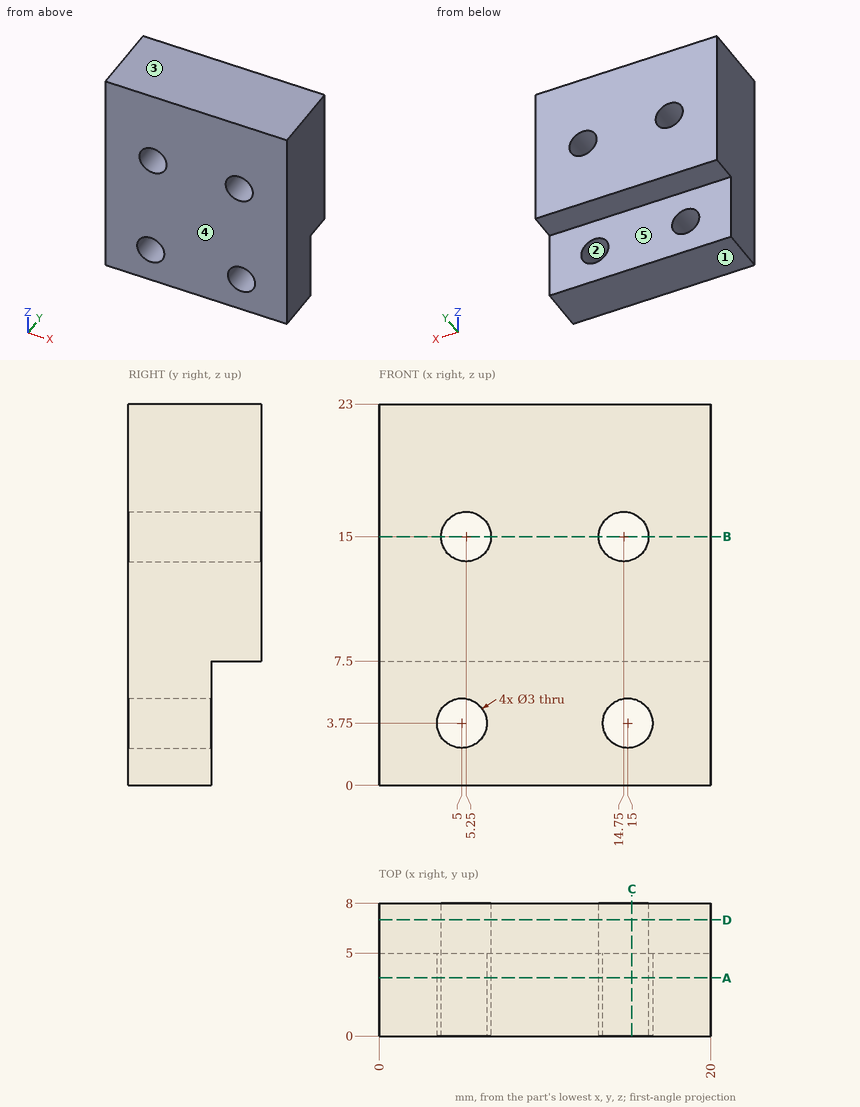
Answer from the drawing. Dimensions are ordinates in mm from the lowest x, y and z of the part. A direction names the side the tool comes from. Coordinates: 2 decimals unless noted, no trailing zeros. Loops run counter-clockwise (first coordinate to the right, second up) from the corner with the lowest first, then second, coordinate; pieces in that order, holes last. Notation, with made-up numbers: (60.25, 29.5) - (78.25, 29.5) arc R14 ccw to (78.25, 34.5) - close; hole circle Ø6 at (-22.5, 83). An arc over 180 degrees is marked (long way). Use a Markdown table: item, result.
Item 1: Find section C-C, the plane x = 15.25. Determine the outline of the cut face in (y, z), and give its area (3 significant figures).
Evaluation:
| item | result |
|---|---|
| outline | (0, 0) - (5, 0) - (5, 2.27) - (0, 2.27) - close; (0, 5.23) - (5, 5.23) - (5, 7.5) - (8, 7.5) - (8, 13.59) - (0, 13.59) - close; (0, 16.41) - (8, 16.41) - (8, 23) - (0, 23) - close |
| area | 124 mm2 |
Item 2: Find section D-D, the plane y = 7. Determine the outline of the cut face in (x, z), and give its area (3 significant figures).
Evaluation:
| item | result |
|---|---|
| outline | (0, 7.5) - (20, 7.5) - (20, 23) - (0, 23) - close; hole circle Ø3 at (5.25, 15); hole circle Ø3 at (14.75, 15) |
| area | 296 mm2 |
Item 3: Find section B-B, the plane z = 15. Determine the outline of the cut face in (x, y).
Evaluation:
| item | result |
|---|---|
| outline | (0, 0) - (3.75, 0) - (3.75, 8) - (0, 8) - close; (6.75, 0) - (13.25, 0) - (13.25, 8) - (6.75, 8) - close; (16.25, 0) - (20, 0) - (20, 8) - (16.25, 8) - close |
Item 4: For the marked faces 4 and 5, determine the directions among +Z, -Z, +X, -X, +Y, -Y from which every point of the face is accessible in a straight line to the end or side of a thin tool.
Evaluation:
| item | result |
|---|---|
| face 4 | +Z, -Z, +X, -X, -Y |
| face 5 | -Z, +X, -X, +Y |
Item 5: The mould has two halves that part along Z. Classify the marked faces 1, 2 and 3: +Z half, -Z half, draft (parallel to the pull), parting line (faces both ways), or undercut.
Evaluation:
| item | result |
|---|---|
| face 1 | -Z half |
| face 2 | undercut |
| face 3 | +Z half |
Item 6: Find section A-A, the plane y = 3.5. Determine the outline of the cut face in (x, z).
Evaluation:
| item | result |
|---|---|
| outline | (0, 0) - (20, 0) - (20, 23) - (0, 23) - close; hole circle Ø3 at (5, 3.75); hole circle Ø3 at (5.25, 15); hole circle Ø3 at (14.75, 15); hole circle Ø3 at (15, 3.75) |
Item 7: Given pin 1 Ø3 at (x, z) = (3, 9) entering from -Y; pin 2 Ø0.9 at (x, y) = (11, 6.5) entering from -Z; pin 3 Ø2.5 at (x, z) = (5, 3.75) entering from -Y; pin 4 Ø5 at (x, z) = (15, 3.75) entering from +Y, each flat-ended and moving along its own axis, determine where each tip first touches the part or whether it passes through.
Evaluation:
| item | result |
|---|---|
| pin 1 | stops at y = 0 |
| pin 2 | stops at z = 7.5 |
| pin 3 | passes through |
| pin 4 | stops at y = 5 |
Item 8: Consider probe 1 along X at (y, z) = (5, 15); probe 2 along X at (y, z) = (2.85, 3.75); probe 3 along Z at (x, y) = (5.25, 5.5). Determine where each line is inside the solid, lowest interval first. Write a range as from..to.
Evaluation:
| item | result |
|---|---|
| probe 1 | x = 0..3.75, 6.75..13.25, 16.25..20 |
| probe 2 | x = 0..3.5, 6.5..13.5, 16.5..20 |
| probe 3 | z = 7.5..13.5, 16.5..23 |
